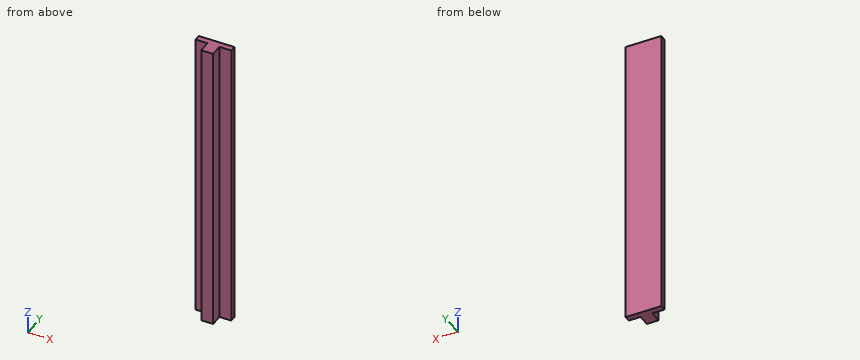
```python
from build123d import *

# Parameters (mm, degrees)
F0_W     = 2
F0_H     = 2
F0_W_2   = 4
F1_DEPTH = 50


with BuildPart() as f1:
    # F0 (on Top) → F1 (new body, symmetric)
    with BuildSketch(Plane.XY):
        with Locations((-1, 5)):
            Rectangle(F0_W, F0_H)
        with Locations((1, 5)):
            Rectangle(F0_W, F0_H)
        with Locations((4, 5)):
            Rectangle(F0_W_2, F0_H)
        Polygon((-2, 4), (-2, 0), (2, 0), (2, 4), (0, 4), align=None)
        with Locations((-4, 5)):
            Rectangle(F0_W_2, F0_H)
    extrude(amount=F1_DEPTH, both=True)


solid = f1.part
```
Model file for the job. Use its own axes, mm. Round coordinates to 2 decimals unless told otherwise and drop trailing zeros. Write each loop counter-clockwise with the first axis right and the second up, starting at its lowest first coordinate (ties: lowest second). Pieces come first, ordered by that corner, then holes. Notation, with made-up numbers: (26.5, 68.5) - (31.5, 68.5) arc R29 ccw to (31.5, 101.5) - close; hole circle Ø2 at (61, 72). An arc over 180 degrees is marked (long way). Use CSV: the item, a comma, the result in double quotes. Start each with the question number.
Item 1: Pin check, flat tips, straight feed: P1, Ø3, axis at x = 4, z = -18, coming from the -Y side; P2, Ø2, axis at y = 1.5, z = -3, coming from the -X side; P3, Ø1.5, axis at y = 1.5, z = 24.5, coming from the +X side. Stop position of each tip, or through.
Item 2: Band-saw the part on A-A (z = 20). Write the cut outline in (x, y).
Item 3: Drill centre lines: L1, parallel to Y at x = 2.75, z = 16; L2, parallel to X at y = 0.7, z = -12.5. Where is each one in solid material? Low to high. Write a range as [from, to].
Item 4: Band-saw the part on B-B (x = 4.5). Write the cut outline in (y, z).
Item 5: Band-saw the part on C-C (y = 1.45). Write the cut outline in (x, z), and give its area (3 significant figures).
Checked values:
1,P1,"stops at y = 4"
1,P2,"stops at x = -2"
1,P3,"stops at x = 2"
2,outline,"(-6, 4) - (-2, 4) - (-2, 0) - (2, 0) - (2, 4) - (6, 4) - (6, 6) - (-6, 6) - close"
3,L1,"y = [4, 6]"
3,L2,"x = [-2, 2]"
4,outline,"(4, -50) - (6, -50) - (6, 50) - (4, 50) - close"
5,outline,"(-2, -50) - (2, -50) - (2, 50) - (-2, 50) - close"
5,area,"400 mm²"
